from build123d import *

# Parameters (mm, degrees)
SKETCH1_W           = 38.65
SKETCH1_H           = 23
BOSS_EXTRUDE1_DEPTH = 31.5
CUT_EXTRUDE1_DEPTH  = 20
SKETCH4_R           = 0.8
CUT_EXTRUDE2_DEPTH  = 2.15
BOSS_EXTRUDE2_START = -6
SKETCH7_W           = 10
SKETCH7_H           = 23
SKETCH7_R           = 1.5
SKETCH7_W_2         = 37.65
SKETCH7_H_2         = 8
BOSS_EXTRUDE2_DEPTH = 7.5


with BuildPart() as part:
    # Sketch1 → Boss-Extrude1 (new body)
    with BuildSketch(Plane(origin=(0, 0, 0), x_dir=(1, 0, 0), z_dir=(0, 1, 0))):
        with Locations((19.325, 11.5)):
            Rectangle(SKETCH1_W, SKETCH1_H)
    extrude(amount=BOSS_EXTRUDE1_DEPTH)

    # Sketch3 → Cut-Extrude1 (cut)
    with BuildSketch(Plane.XY):
        Polygon((2, 25.5), (2, 6), (4, 6), (4, 3), (36.5, 3), (36.5, 8.2), (37.65, 8.2), (37.65, 23.3), (36.5, 23.3), (36.5, 28.5), (4, 28.5), (4, 25.5), align=None)
    extrude(amount=-CUT_EXTRUDE1_DEPTH, mode=Mode.SUBTRACT)

    # Sketch4 → Cut-Extrude2 (cut)
    with BuildSketch(Plane.ZY.offset(-36.5)):
        with Locations((-14, 26.55)):
            Circle(SKETCH4_R)
        with Locations((-14, 6.05)):
            Circle(SKETCH4_R)
    extrude(amount=-CUT_EXTRUDE2_DEPTH, mode=Mode.SUBTRACT)

    # Sketch7 → Boss-Extrude2 (add)
    # profile 1 of 2: a face of its own
    with BuildSketch(Plane.XZ.offset(BOSS_EXTRUDE2_START)):
        with Locations((-5, -11.5)):
            Rectangle(SKETCH7_W, SKETCH7_H)
        with Locations(Location((-5, -17.5, 0), (0, 0, 270))):
            Circle(SKETCH7_R, mode=Mode.SUBTRACT)
        with Locations(Location((-5, -5.5, 0), (0, 0, 270))):
            Circle(SKETCH7_R, mode=Mode.SUBTRACT)
    # profile 2 of 2: a face of its own
    with BuildSketch(Plane.XZ.offset(BOSS_EXTRUDE2_START)):
        with Locations((19.825, -27)):
            Rectangle(SKETCH7_W_2, SKETCH7_H_2)
        with Locations(Location((30.65, -27, 0), (0, 0, 270))):
            Circle(SKETCH7_R, mode=Mode.SUBTRACT)
        with Locations(Location((9, -27, 0), (0, 0, 270))):
            Circle(SKETCH7_R, mode=Mode.SUBTRACT)
    extrude(amount=-BOSS_EXTRUDE2_DEPTH)


solid = part.part
Geometry: final body of the model. Coordinates: model frame, mm. A direction names the side the tool comes from. Coordinates: 2 decimals unless noted, no trailing zeros. Loops run counter-clockwise (first coordinate to the right, second up) from the corner with the lowest first, then second, coordinate; pieces in that order, holes last. Notation, with made-up numbers: (45, 22.5) - (101, 22.5) arc R16 cw to (101, 36.5) - close; hole circle Ø10 at (22.25, 18.25). An arc over 180 degrees is marked (long way). Put each result on its own line as item: value. Start each with the question number.
Q1. Pull-direction query (Y, two-part tool) for faces 5 (the flat face through (19, 0, -12)), 6 (the flat face through (4, 5, -10)), 7 (the flat face through (20, 10, -31)); classes: released by +Y, released by -Y, zero draft, split by the parting line, or undercut.
Q2. Cut plane C-C, the plane x = 9. Return loops of the section in (y, z), and give its area (3 significant figures).
Q3. Pin query (flat end, axial travel): pin 1 Ø4 at (y, z) = (10, -27) entering from -X; pin 2 Ø5 at (y, z) = (1.5, -8) entering from -X; pin 3 Ø4 at (x, z) = (9, -27) entering from -Y. Return the tip coordinate at first contact, or that it passes through.
Q4. Line query: line 1 (Y direction, x = 37.95, z = -14); line 2 (Y direction, x = 37, z = -14); line 3 (X direction, y = 9, z = -27). Output: solid intervals per line, ascending.
Q5. Cut plane B-B, the plane x = -5. Return loops of the section in (y, z).
Q6. Cut plane D-D, the plane z = -14. Return loops of the section in (x, y), and give its area (3 significant figures).
Q7. Set-up query: faces 1 (the flat face through (20, 6, -27)), 2 (the flat face through (20, 13.5, -27)), 3 (the flat face through (37, 23.3, -10)), 4 (the flat face through (-5, 13.5, -11)). Return all of +Z, -Z, +X, -X, +Y, -Y with unobstructed straight access to the full face (end or side cutting, diameter ignored); none if empty.
Q8. Cut plane A-A, the plane z = -17.5. Return loops of the section in (x, y).
Filled sheet:
1. face 5: released by -Y
1. face 6: undercut
1. face 7: zero draft
2. outline: (0, -23) - (6, -23) - (6, -25.5) - (13.5, -25.5) - (13.5, -23) - (31.5, -23) - (31.5, 0) - (28.5, 0) - (28.5, -20) - (3, -20) - (3, 0) - (0, 0) - close; (6, -31) - (13.5, -31) - (13.5, -28.5) - (6, -28.5) - close
2. area: 252 mm²
3. pin 1: x = 1
3. pin 2: x = 0
3. pin 3: y = 6
4. line 1: 0 to 5.25, 6.85 to 25.75, 27.35 to 31.5
4. line 2: 0 to 5.25, 6.85 to 8.2, 23.3 to 25.75, 27.35 to 31.5
4. line 3: 1 to 7.5, 10.5 to 29.15, 32.15 to 38.65
5. outline: (6, -23) - (13.5, -23) - (13.5, -19) - (6, -19) - close; (6, -16) - (13.5, -16) - (13.5, -7) - (6, -7) - close; (6, -4) - (13.5, -4) - (13.5, 0) - (6, 0) - close
6. outline: (-10, 6) - (0, 6) - (0, 0) - (38.65, 0) - (38.65, 5.25) - (36.5, 5.25) - (36.5, 3) - (4, 3) - (4, 6) - (2, 6) - (2, 25.5) - (4, 25.5) - (4, 28.5) - (36.5, 28.5) - (36.5, 27.35) - (38.65, 27.35) - (38.65, 31.5) - (0, 31.5) - (0, 13.5) - (-10, 13.5) - close; (36.5, 6.85) - (38.65, 6.85) - (38.65, 25.75) - (36.5, 25.75) - (36.5, 23.3) - (37.65, 23.3) - (37.65, 8.2) - (36.5, 8.2) - close
6. area: 400 mm²
7. face 1: -Z, +X, -X, -Y
7. face 2: -Z, +X, -X, +Y
7. face 3: +Z
7. face 4: +Z, -Z, -X, +Y
8. outline: (-10, 6) - (-6.5, 6) - (-6.5, 13.5) - (-10, 13.5) - close; (-3.5, 6) - (0, 6) - (0, 0) - (38.65, 0) - (38.65, 31.5) - (0, 31.5) - (0, 13.5) - (-3.5, 13.5) - close; hole (2, 6) - (4, 6) - (4, 3) - (36.5, 3) - (36.5, 8.2) - (37.65, 8.2) - (37.65, 23.3) - (36.5, 23.3) - (36.5, 28.5) - (4, 28.5) - (4, 25.5) - (2, 25.5) - close
